Autodesk Inventor part; units mm, degrees
ref_plane "YZ Plane" through (0, 0, 0) normal (1, 0, 0) x (0, 1, 0)
ref_plane "XZ Plane" through (0, 0, 0) normal (0, 1, 0) x (-1, 0, 0)
ref_plane "XY Plane" through (0, 0, 0) normal (0, 0, 1) x (1, 0, 0)
sketch "Sketch1" plane through (0, 0, 0) normal (0, 1, 0) x (-1, 0, 0)
  line L0 (0, 0) -> (76.2, 0)
  line L1 (76.2, 0) -> (76.2, -254)
  line L2 (76.2, -254) -> (0, -254)
  line L3 (0, -254) -> (0, 0)
  dimension "d0" = 254
  dimension "d1" = 76.2
extrude "Extrusion1" add sketch "Sketch1" along normal blind 19.05
sketch "Sketch2" plane through (0, 19.05, 0) normal (0, 1, 0) x (1, 0, 0)
  line L0 (-76.2, 0) -> (0, 0)
  line L1 (-49.2125, 0) -> (-49.2125, 850.9)
  line L2 (0, 0) -> (0, 254)
  line L3 (-76.2, 254) -> (-76.2, 0)
  circle A0 centre (-49.2125, 50.8) radius 4.7625
  circle A1 centre (-49.2125, 93.6625) radius 4.7625
  circle A2 centre (-49.2125, 136.525) radius 4.7625
  circle A3 centre (-49.2125, 179.3875) radius 4.7625
  circle A4 centre (-49.2125, 222.25) radius 4.7625
  dimension "d4" = 26.9875
  dimension "d5" = 50.8
  dimension "d6" = 9.525
  dimension "d7" = 42.8625
  dimension "d8" = 42.8625
  dimension "d9" = 42.8625
  dimension "d10" = 42.8625
extrude "Extrusion2" cut sketch "Sketch2" against normal up to surface (19.05 mm away)
equation "\"d0\" = botPlateLength"
equation "\"d1\" = botPlateWidth"
equation "\"d2\" = woodThickness"
equation "\"d4\" = tuningPegOffset"
equation "\"d5\" = tuningPegEndOffset"
equation "\"d6\" = tuningPegDiameter"
equation "\"d7\" = tuningPegSeparation"
equation "\"d8\" = tuningPegSeparation"
equation "\"d9\" = tuningPegSeparation"
equation "\"d10\" = tuningPegSeparation"
equation "\"botPlateWidth\" = 76.2"
equation "\"woodThickness\" = 19.05"
equation "\"stringLength\" = 647.7"
equation "\"neckLength\" = 203.2"
equation "\"tuningPegOffset\" = 26.9875"
equation "\"tuningPegDiameter\" = 9.525"
equation "\"tuningPegEndOffset\" = 50.8"
properties part number "bodyBotPlate"
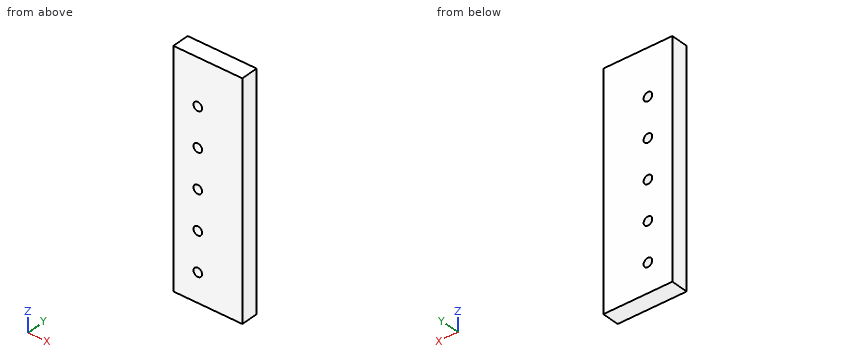
Here's how the part is built. I have some questions about the finished solid (model axes, mm). Coordinates: 2 decimals unless noted, no trailing zeros. Order: outer loops, then holes, each group sorted by start corner. A loop starts at its lowest first (then second) coordinate and runs counter-clockwise, first axis right, second up.
1) Imagine slicing it at A-A on z = -222.25. List the corners of the cut face in (x, y) for me (3 decimals).
2) Imagine slicing it at B-B on y = 5. State how many separate pieces and enclosed holes the cut face has, and give its area (3 significant figures).
3) I need wall thicknesses on line 1 (X direction, y = 13.25, z = -50.8) (3 decimals); line 2 (Z direction, x = -49.5, y = 2.25); line 3 (Z direction, x = -53.5, y = 12.5). Which ranges of each line are inside material? Lowest first, please.
Response values:
1. outline: (-76.2, 0) - (-53.975, 0) - (-53.975, 19.05) - (-76.2, 19.05) - close; (-44.45, 0) - (0, 0) - (0, 19.05) - (-44.45, 19.05) - close
2. separate pieces: 1
2. enclosed holes: 5
2. area: 19,000 mm2
3. line 1: x = -76.2 to -53.975, -44.45 to 0
3. line 2: z = -254 to -227, -217.5 to -184.14, -174.63 to -141.28, -131.77 to -98.42, -88.91 to -55.55, -46.05 to 0
3. line 3: z = -254 to -224.32, -220.18 to -181.46, -177.31 to -138.6, -134.45 to -95.74, -91.59 to -52.87, -48.73 to 0
